Input: part model. Units: mm. Frame: model coordinates. Round coordinates to 2 decimals unless told otherwise and drop trailing zeros. Order: outer loops, then holes, each group sorted by start corner. A loop starts at its lowest first (then second) coordinate and runs counter-clockwise, first axis right, second up.
Item 1: Cut plane B-B on x = 2.25. Output: boundary loops of the cut face in (y, z), then the cut area to 3 significant figures.
Item 2: Cut plane A-A on y = -1.7. Output: boundary loops of the cut face in (x, z), then the cut area to 3 significant figures.
Item 3: Line query: L1, parallel to X at y = -1, z = 0.1; L2, parallel to X at y = -1.35, z = 0.25; L3, parallel to Z at x = 4.5, y = -0.7. Output: solid intervals per line, ascending.
Item 4: Cut plane C-C on z = 0.25. Output: boundary loops of the cut face in (x, y).
Item 5: First-contact query: pin 1 (0.8 mm diameter, centred on y = -2, z = 0.5, fed in from -X); pin 2 (0.7 mm diameter, centred on x = 6, z = -1, fed in from -Y); pin 3 (0.5 mm diameter, centred on x = 5.5, z = 1.5, fed in from -Y). Flat tips, straight axial feed; report the tip coordinate or a pass-through.
Item 6: Cut plane D-D on y = -1.3. Output: boundary loops of the cut face in (x, z).
Item 7: Mould query, pull axis Z, two halves, no side actions, for faces 1 (the cylindrical face through (3.894, -1.345, 1.741)), 2 (the flat face through (-0.298, -1.173, -0.03)), 3 (the flat face through (8, -1, 0)), 4 (the flat face through (1, -1, 0)). Classes: released by +Z, released by -Z, zero draft, split by the parting line, or undercut.
```python
from build123d import *

# Parameters (mm, degrees)
BOX003_W               = 14
BOX003_H               = 10
BOX003_DEPTH           = 10
BOX003_PLACEMENT_ANGLE = 60
BOX002_W               = 7
BOX002_H               = 1.6
BOX002_DEPTH           = 3
BOX001_W               = 7
BOX001_H               = 5
BOX001_DEPTH           = 1.7
BOX_W                  = 14
BOX_H                  = 7
BOX_DEPTH              = 10
CYLINDER_R             = 2.2
CYLINDER_DEPTH         = 13


with BuildPart() as obj1:
    # Box003 → Box003 (new body)
    with BuildSketch(Plane.XY):
        with Locations((7, 5)):
            Rectangle(BOX003_W, BOX003_H)
    extrude(amount=BOX003_DEPTH)


with BuildPart() as obj1_1:
    # Box003 placement: moved
    add(obj1.part.moved(Location((-3.2, -6.2, -4))).rotate(Axis((-3.2, -6.2, -4), (0, 0, 1)), BOX003_PLACEMENT_ANGLE))


with BuildPart() as obj2:
    # Box002 → Box002 (new body)
    with BuildSketch(Plane(origin=(1, -2.6, -1.5), x_dir=(1, 0, 0), z_dir=(0, 0, 1))):
        with Locations((3.5, 0.8)):
            Rectangle(BOX002_W, BOX002_H)
    extrude(amount=BOX002_DEPTH)


with BuildPart() as obj3:
    # Box001 → Box001 (new body)
    with BuildSketch(Plane(origin=(1, -4, -0.85), x_dir=(1, 0, 0), z_dir=(0, 0, 1))):
        with Locations((3.5, 2.5)):
            Rectangle(BOX001_W, BOX001_H)
    extrude(amount=BOX001_DEPTH)


with BuildPart() as obj4:
    # Box → Box (new body)
    with BuildSketch(Plane(origin=(-4, -0.5, -4), x_dir=(1, 0, 0), z_dir=(0, 0, 1))):
        with Locations((7, 3.5)):
            Rectangle(BOX_W, BOX_H)
    extrude(amount=BOX_DEPTH)


with BuildPart() as body:
    # Sketch → Revolution (revolve)
    with BuildSketch(Plane.XY):
        with BuildLine():
            add(Edge.make_bspline(
                [(1.699821, 2.2), (2.24, 1.1), (2.24, 0)],
                knots=[-2.2, -2.2, -2.2, 0, 0, 0], degree=2))
            Line((2.24, 0), (1.699821, 0))
            Line((1.699821, 0), (1.699821, 2.2))
        make_face()
    revolve(axis=Axis((0, 0, 0), (1, 0, 0)))


with BuildPart() as body_1:
    # Body placement: moved
    add(body.part.moved(Location((-1.7, 20, 0))))


with BuildPart() as cut004:
    # Cylinder → Cylinder (new body)
    with BuildSketch(Plane(origin=(-4, 0, 0), x_dir=(0, 0, -1), z_dir=(1, 0, 0))):
        Circle(CYLINDER_R)
    extrude(amount=CYLINDER_DEPTH)

    # Cut: cut Body
    add(body_1.part, mode=Mode.SUBTRACT)

    # Cut001: cut obj4
    add(obj4.part, mode=Mode.SUBTRACT)

    # Cut002: cut obj3
    add(obj3.part, mode=Mode.SUBTRACT)

    # Cut003: cut obj2
    add(obj2.part, mode=Mode.SUBTRACT)

    # Cut004: cut obj1
    add(obj1_1.part, mode=Mode.SUBTRACT)


solid = cut004.part
```
From the geometry:
1. outline: (-1.61, -1.5) arc R2.2 ccw to (-0.5, -2.14) - (-0.5, -0.85) - (-1, -0.85) - (-1, -1.5) - close; (-1.61, 1.5) - (-1, 1.5) - (-1, 0.85) - (-0.5, 0.85) - (-0.5, 2.14) arc R2.2 ccw to start
1. area: 1.53 mm2
2. outline: (-0.6, -1.4) - (1, -1.4) - (1, 1.4) - (-0.6, 1.4) - close; (8, -1.4) - (9, -1.4) - (9, 1.4) - (8, 1.4) - close
2. area: 7.27 mm2
3. L1: x = -0.2 to 1, 8 to 9
3. L2: x = -0.4 to 1, 8 to 9
3. L3: z = -2.09 to -0.85, 0.85 to 2.09
4. outline: (-0.88, -2.19) - (1, -2.19) - (1, -0.5) - (0.09, -0.5) - close; (8, -2.19) - (9, -2.19) - (9, -0.5) - (8, -0.5) - close
5. pin 1: stops at x = -0.89
5. pin 2: stops at y = -1
5. pin 3: stops at y = -1.61
6. outline: (-0.37, -1.77) - (9, -1.77) - (9, 1.77) - (-0.37, 1.77) - close; hole (1, -1.5) - (8, -1.5) - (8, 1.5) - (1, 1.5) - close
7. face 1: split by the parting line
7. face 2: zero draft
7. face 3: undercut
7. face 4: undercut
